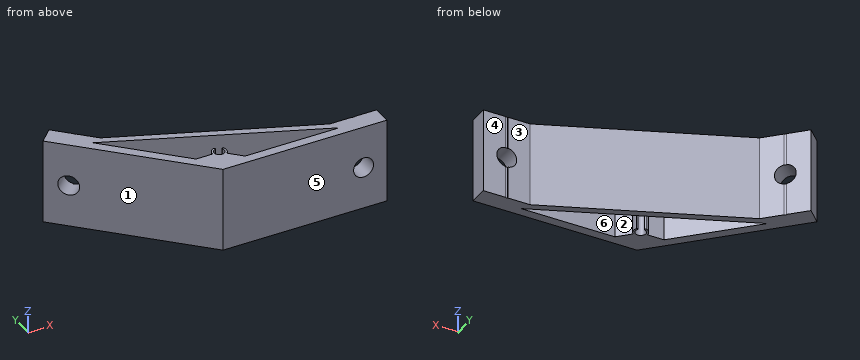
from build123d import *

# Parameters (mm, degrees)
EXTRUDE_1_DEPTH                 = 36
CUT_EXTRUDE_1_REACH             = 93.758
SKETCH_2_R                      = 4.25
CUT_EXTRUDE_2_REACH             = 90.803
SKETCH_3_R                      = 4.25
CUT_EXTRUDE_2_DIRECTION_2_DEPTH = 89.803380595
SKETCH_4_W                      = 1
SKETCH_4_H                      = 36
CUT_EXTRUDE_3_DEPTH             = 0.2
SKETCH_5_W                      = 36
SKETCH_5_H                      = 1
CUT_EXTRUDE_4_DEPTH             = 0.2


with BuildPart() as part:
    # 草图1 → 凸台-拉伸1 (new body)
    with BuildSketch(Plane.XY):
        Polygon((0, 0), (70, 0), (70, 8), (50, 8), (-29.69848481, 41.012193309), (-43.840620434, 55.154328933), (-49.497474683, 49.497474683), align=None)
        with BuildLine():
            Line((-33.812061864, 39.468916114), (-5.414213562, 11.071067812))
            Line((-5.414213562, 11.071067812), (1.735433814, 11.071067812))
            ThreePointArc((1.735433814, 11.071067812), (2.215643659, 13.045304249), (3.843807178, 14.260744318))
            ThreePointArc((3.843807178, 14.260744318), (4.355517598, 13.988067869), (4.08284115, 13.476357449))
            ThreePointArc((4.08284115, 13.476357449), (3.884071826, 9.376978879), (6.642219074, 12.416228401))
            ThreePointArc((6.642219074, 12.416228401), (6.811241616, 12.970873675), (7.365886891, 12.801851133))
            ThreePointArc((7.365886891, 12.801851133), (7.657726441, 10.791119753), (6.601290107, 9.055564143))
            Line((6.601290107, 9.055564143), (11.656854249, 4))
            Line((11.656854249, 4), (51.81747646, 4))
            Line((51.81747646, 4), (-33.812061864, 39.468916114))
        make_face(mode=Mode.SUBTRACT)
    extrude(amount=EXTRUDE_1_DEPTH)

    # 草图2 → 切除-拉伸1 (cut, up to next)
    with BuildSketch(Plane(origin=(0, 8, 0), x_dir=(1, 0, 0), z_dir=(0, 1, 0)), mode=Mode.PRIVATE) as cut_extrude_1_sk1:
        with Locations(Location((60, -18, 0), (0, 0, 270))):
            Circle(SKETCH_2_R)
    cut_extrude_1_tool1 = extrude(cut_extrude_1_sk1.sketch, amount=-CUT_EXTRUDE_1_REACH, mode=Mode.PRIVATE) & part.part
    add(cut_extrude_1_tool1.solids().sort_by_distance((60, 8, 18))[0], mode=Mode.SUBTRACT)

    # 草图3 → 切除-拉伸2 (cut, up to next)
    with BuildSketch(Plane(origin=(5.656854249, 5.656854249, 0), x_dir=(0, 0, -1), z_dir=(0.7071067811865437, 0.7071067811865513, 0)), mode=Mode.PRIVATE) as cut_extrude_2_sk1:
        with Locations(Location((-18, 60, 0), (0, 0, 270))):
            Circle(SKETCH_3_R)
    cut_extrude_2_tool1 = extrude(cut_extrude_2_sk1.sketch, amount=-CUT_EXTRUDE_2_REACH, mode=Mode.PRIVATE) & part.part
    add(cut_extrude_2_tool1.solids().sort_by_distance((-36.769553, 48.083261, 18))[0], mode=Mode.SUBTRACT)

    # 草图3 → 切除-拉伸2 direction 2 (cut)
    with BuildSketch(Plane(origin=(5.656854249, 5.656854249, 0), x_dir=(0, 0, -1), z_dir=(0.7071067811865437, 0.7071067811865513, 0))):
        with Locations(Location((-18, 60, 0), (0, 0, 270))):
            Circle(SKETCH_3_R)
    extrude(amount=CUT_EXTRUDE_2_DIRECTION_2_DEPTH, mode=Mode.SUBTRACT)

    # 草图4 → 切除-拉伸3 (cut)
    with BuildSketch(Plane(origin=(0, 8, 0), x_dir=(1, 0, 0), z_dir=(0, 1, 0))):
        with Locations((60, -18)):
            Rectangle(SKETCH_4_W, SKETCH_4_H)
    extrude(amount=-CUT_EXTRUDE_3_DEPTH, mode=Mode.SUBTRACT)

    # 草图5 → 切除-拉伸4 (cut)
    with BuildSketch(Plane(origin=(5.656854249, 5.656854249, 0), x_dir=(0, 0, -1), z_dir=(0.7071067811865437, 0.7071067811865513, 0))):
        with Locations((-18, 60)):
            Rectangle(SKETCH_5_W, SKETCH_5_H)
    extrude(amount=-CUT_EXTRUDE_4_DEPTH, mode=Mode.SUBTRACT)


solid = part.part
Read the model definition and answer for the solid it produces. Units are mm, in the model's axes. Face numbers are marked on the shaded views. A direction names the side the tool comes from. Give positions to 0.01 mm unless a question says otherwise; leave off trailing zeros. Write each loop counter-clockwise with the first axis right and the second up, starting at its lowest first coordinate (ties: lowest second). Pieces come first, ordered by that corner, then holes. Notation, with made-up numbers: (52, -11) - (76, -11) arc R18 cw to (76, 16) - close; hole circle Ø4 at (-20, 21.5). An arc over 180 degrees is marked (long way). Use CSV: the item, a comma, the result in double quotes. Start each with the question number.
(1) Given P1, Ø8, axis at x = -18, z = 20, coming from the +Y side; P2, Ø8, axis at x = 9.5, z = 15.5, coming from the +Y side; P3, Ø11, axis at x = 60, z = 18, coming from the +Y side; P4, Ø5.5, axis at x = 4.72, y = 11.39, coming from the -Z side, each flat-ended and moving along its own axis, determine where each tip first touches the part or whether it passes through.
(2) Determine the mould class of the marked faces 1, 2 and 3 for opening direction Y: +Y half, -Y half, draft (parallel to the pull), parting line (faces both ways), or undercut.
(3) Find section B-B (x = -21.5). Give the vertices of the cut face in (y, z), plus the area to 3 significant figures.
(4) For the marked faces 4, 5 and 6, determine the directions among +Z, -Z, +X, -X, +Y, -Y from which every point of the face is accessible in a straight line to the end or side of a thin tool.
(5) Find section D-D (z = 10). Give the vertices of the cut face in (x, y), plus the area to 3 significant figures.
(6) Consider line 1 along X through (y, z) = (4.25, 18); line 2 along Z through (x, y) = (60, 5); line 3 along X through (y, z) = (6, 20.5). Determine where each line is inside the solid, lowest interval first.
(7) Find section C-C (y = 31). Give the vertices of the cut face in (x, z).
(8) Find section A-A (z = 20.5). Give the vertices of the cut face in (x, y), plus the area to 3 significant figures.
Findings below:
1,P1,"y = 37.82"
1,P2,"y = 26.43"
1,P3,"y = 8"
1,P4,"z = 0"
2,face 1,"-Y half"
2,face 2,"undercut"
2,face 3,"+Y half"
3,outline,"(21.5, 0) - (27.16, 0) - (27.16, 36) - (21.5, 36) - close; (34.37, 0) - (37.62, 0) - (37.62, 36) - (34.37, 36) - close"
3,area,"321 mm2"
4,face 4,"+Z, -Z, +X, +Y"
4,face 5,"+Z, -Z, +X, -X, -Y"
4,face 6,"+Z, -Z"
5,outline,"(-49.5, 49.5) - (0, 0) - (70, 0) - (70, 8) - (60.5, 8) - (60.5, 7.8) - (59.5, 7.8) - (59.5, 8) - (50, 8) - (-29.7, 41.01) - (-36.42, 47.73) - (-36.56, 47.59) - (-37.26, 48.3) - (-37.12, 48.44) - (-43.84, 55.15) - close; hole (-33.81, 39.47) - (-5.41, 11.07) - (1.74, 11.07) arc R3 cw to (3.84, 14.26) arc R0.41 cw to (4.08, 13.48) arc R2.18 ccw (long way) to (6.64, 12.42) arc R0.41 cw to (7.37, 12.8) arc R3 cw to (6.6, 9.06) - (11.66, 4) - (51.82, 4) - close"
5,area,"1,050 mm2"
6,line 1,"-4.25 to 11.41, 51.21 to 55.75, 64.25 to 70"
6,line 2,"0 to 13.75, 22.25 to 36"
6,line 3,"-6 to 9.66, 46.99 to 56.56, 63.44 to 70"
7,outline,"(-31, 0) - (-25.34, 0) - (-25.34, 36) - (-31, 36) - close; (-13.37, 0) - (-5.53, 0) - (-5.53, 36) - (-13.37, 36) - close"
8,outline,"(-49.5, 49.5) - (-44.86, 44.86) - (-39.2, 50.51) - (-43.84, 55.15) - close; (-40, 40) - (0, 0) - (56.56, 0) - (56.56, 8) - (50, 8) - (-29.7, 41.01) - (-34.34, 45.65) - close; (63.44, 0) - (70, 0) - (70, 8) - (63.44, 8) - close; hole (-33.81, 39.47) - (-5.41, 11.07) - (1.74, 11.07) arc R3 cw to (3.84, 14.26) arc R0.41 cw to (4.08, 13.48) arc R2.18 ccw (long way) to (6.64, 12.42) arc R0.41 cw to (7.37, 12.8) arc R3 cw to (6.6, 9.06) - (11.66, 4) - (51.82, 4) - close"
8,area,"937 mm2"
